The model under review builds one solid part; all positions refer to its coordinate system, in mm. Round coordinates to 2 decimals unless told otherwise and drop trailing zeros. Write each loop counter-clockwise with the first axis right and the second up, starting at its lowest first coordinate (ties: lowest second). Pieces come first, ordered by that corner, then holes. Notation, with made-up numbers: (40.25, 74) - (61.25, 74) arc R9 ccw to (61.25, 89) - close; hole circle Ø4 at (28, 23). An arc over 180 degrees is marked (long way). Use one line per item in the form item = value.
Autodesk Inventor part; units mm, degrees
ref_plane "YZ Plane" through (0, 0, 0) normal (1, 0, 0) x (0, 1, 0)
ref_plane "XZ Plane" through (0, 0, 0) normal (0, 1, 0) x (-1, 0, 0)
ref_plane "XY Plane" through (0, 0, 0) normal (0, 0, 1) x (1, 0, 0)
sketch "Sketch1" plane through (0, 0, 0) normal (0, 1, 0) x (-1, 0, 0)
  arc A0 (2.9205, -0.0553) -> (-2.9205, -0.0553) centre (0, 0) ccw
  arc A1 (-1.5, -150) -> (1.5, -150) centre (0, -150) ccw
  line L0 (2.921, 0) -> (1.5, -150)
  line L1 (-2.921, 0) -> (-1.5, -150)
  dimension "d1" = 5.842
  dimension "d3" = 3
extrude "Extrusion1" add sketch "Sketch1" along normal blind 3
sketch "Sketch2" plane through (0, 3, 0) normal (0, 1, 0) x (1, 0, 0)
  circle A0 centre (0, 0) radius 1.905
  dimension "d6" = 3.81
extrude "Extrusion2" cut sketch "Sketch2" against normal blind 3
sketch "Sketch3" plane through (0, 3, 0) normal (0, 1, 0) x (1, 0, 0)
  circle A0 centre (0, 7.62) radius 0.381
  point P0 (0, 0)
  dimension "d10" = 0.762
extrude "Extrusion3" cut sketch "Sketch3" against normal blind 3
properties part number "arm" material "Wood (Cherry)"
(1) Add section C-C on z = -64.5. Write out the cut boundary in (x, y).
Geometry results:
outline = (-2.31, 0) - (2.31, 0) - (2.31, 3) - (-2.31, 3) - close
(2) Add section B-B on z = -109.5. Write out the cut boundary in (x, y).
Geometry results:
outline = (-1.88, 0) - (1.88, 0) - (1.88, 3) - (-1.88, 3) - close
(3) Add section A-A on y = 1.65. Write out the cut boundary in (x, z) (1 decimal).
Geometry results:
outline = (-2.9, -0.1) - (-1.5, -150) arc R1.5 ccw to (1.5, -150) - (2.9, -0.1) arc R2.9 ccw (long way) to start; hole circle Ø3.8 at (0, 0); hole circle Ø0.8 at (0, -7.6)
(4) The part is to be moulded in two halves that separate along X. For faces 1 (the cylindrical face through (0, 1.5, -151.5)), 2 (the cylindrical face through (-0.41, 1.52, 1.86)), 3 (the flat face through (0, 0, -56)), say which applies: +X half, -X half, draft (parallel to the pull), parting line (faces both ways), or undercut.
Geometry results:
face_1 = parting line
face_2 = undercut
face_3 = draft
(5) To check wall thickness, follow L1, parallel to Z at x = 0, y = 0.7 (3 decimals); L2, parallel to X at y = 1.1, z = 0 (3 decimals); L3, parallel to Z at x = -0.3, y = 2.5. State the ranges of each line that lie inside material, in increasing order.
Geometry results:
L1 = -151.5 to -8.001, -7.239 to -1.905, 1.905 to 2.921
L2 = -2.921 to -1.905, 1.905 to 2.921
L3 = -151.47 to -7.85, -7.39 to -1.88, 1.88 to 2.91
(6) Insertion check: P1, Ø3, axis at x = 0, z = 0, coming from the -Y side; P2, Ø1.5, axis at y = 2.5, z = -23, coming from the -X side; P3, Ø1.5, axis at x = 1.5, y = 1, coming from the -Z side; P4, Ø1, axis at y = 2, z = -34.5, coming from the +X side. Each pin has a flat end and moves straight along its axis. Give the tip position at first contact, or say it passes through.
Geometry results:
P1 = through
P2 = -2.71
P3 = -151.3
P4 = 2.6
